The model under review builds one solid part; all positions refer to its coordinate system, in mm. Face numbers are marked on the shaded views. A direction names the side the tool comes from. Coordinates: 2 decimals unless noted, no trailing zeros. Write each loop counter-clockwise with the first axis right and the second up, starting at its lowest first coordinate (ties: lowest second). Pieces come first, ordered by that corner, then holes.
1) Machinability: for the marked faces 1, 2 and 3, which of the approach directions +Z, -Z, +X, -X, +Y, -Y give a long, thin tool a straight path to every point of the face, cutting with its end or side? Answer none if there is none.
2) Add section D-D, the plane y = -7.5. State the section outline as (x, z) points.
3) For P1, Ø5, axis at x = -22.93, y = -0.21, coming from the -Z side; P2, Ø4.5, axis at x = -10.61, y = 10.61, coming from the +Z side; P3, Ø3, axis at x = 20.5, z = 7, coming from the -Y side, all flat-tipped, find the tip position at first contact; note any pin that passes through.
4) Mouldability with a two-part tool opening along X and no side actions: class the marked faces 4, 5, 6 and 7 as released by +X, released by -X, zero draft, split by the parting line, or undercut.
5) Add section B-B, the plane y = 11.5. State the section outline as (x, z) points, then the cut area to 3 significant figures.
6) Add section A-A, the plane x = 0. State the section outline as (y, z) points.
7) Add section C-C, the plane z = 5. Give the number of separate pieces and of enclosed holes in the cut face, then the cut area to 3 significant figures.
8) For line 1 (X direction, y = 14, z = 7.5); line 2 (X direction, y = 0.5, z = 3.5); line 3 (Y direction, x = -13.5, z = 5), list the stretches that pass through material, from the lowest coordinate up.
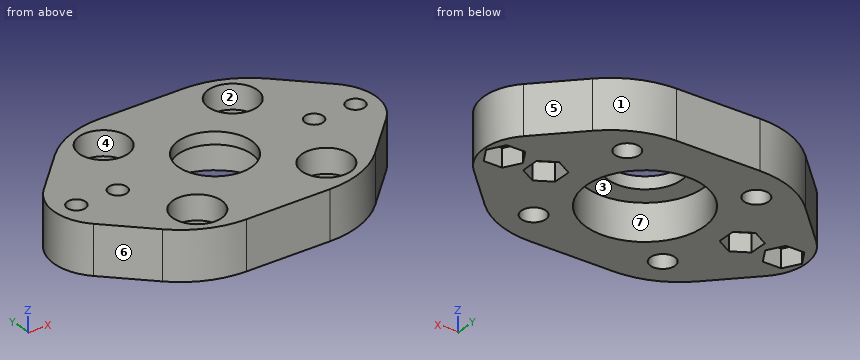
from build123d import *

# Parameters (mm, degrees)
SKETCH1_R           = 2
SKETCH1_R_2         = 9.6
BOSS_EXTRUDE1_DEPTH = 8
SKETCH2_R           = 4
CUT_EXTRUDE1_DEPTH  = 4
SKETCH3_R           = 1.5
CUT_EXTRUDE2_DEPTH  = 10
CUT_EXTRUDE3_DEPTH  = 3
FILLET1_R           = 8
CUT_EXTRUDE4_DEPTH  = 9
FILLET2_R           = 15
SKETCH7_R           = 9.6
SKETCH7_R_2         = 6
BOSS_EXTRUDE2_DEPTH = 2


with BuildPart() as part:
    # Sketch1 → Boss-Extrude1 (new body)
    with BuildSketch(Plane.XY):
        Polygon((-29.69848481, 0), (0, 29.69848481), (29.69848481, 0), (0, -29.69848481), align=None)
        with Locations((10.606601718, 10.606601718)):
            Circle(SKETCH1_R, mode=Mode.SUBTRACT)
        with Locations((10.606601718, -10.606601718)):
            Circle(SKETCH1_R, mode=Mode.SUBTRACT)
        with Locations((-10.606601718, -10.606601718)):
            Circle(SKETCH1_R, mode=Mode.SUBTRACT)
        with Locations((-10.606601718, 10.606601718)):
            Circle(SKETCH1_R, mode=Mode.SUBTRACT)
        Circle(SKETCH1_R_2, mode=Mode.SUBTRACT)
    extrude(amount=BOSS_EXTRUDE1_DEPTH)

    # Sketch2 → Cut-Extrude1 (cut)
    with BuildSketch(Plane.XY.offset(8)):
        with Locations((-10.606601718, 10.606601718)):
            Circle(SKETCH2_R)
        with Locations((10.606601718, 10.606601718)):
            Circle(SKETCH2_R)
        with Locations((10.606601718, -10.606601718)):
            Circle(SKETCH2_R)
        with Locations((-10.606601718, -10.606601718)):
            Circle(SKETCH2_R)
    extrude(amount=-CUT_EXTRUDE1_DEPTH, mode=Mode.SUBTRACT)

    # Sketch3 → Cut-Extrude2 (cut)
    with BuildSketch(Plane.XY.offset(8)):
        with Locations((-22.931196288, -0.213718328)):
            Circle(SKETCH3_R)
        with Locations((-16.131196288, -0.213718328)):
            Circle(SKETCH3_R)
        with Locations((16.131196288, -0.216214782)):
            Circle(SKETCH3_R)
        with Locations((22.931196288, -0.216214782)):
            Circle(SKETCH3_R)
    extrude(amount=-CUT_EXTRUDE2_DEPTH, mode=Mode.SUBTRACT)

    # Sketch4 → Cut-Extrude3 (cut)
    with BuildSketch(Plane(origin=(0, 0, 0), x_dir=(-1, 0, 0), z_dir=(0, 0, -1))):
        Polygon((-24.446740745, 2.408785218), (-25.962285202, -0.216214782), (-24.446740745, -2.841214782), (-21.415651832, -2.841214782), (-19.900107375, -0.216214782), (-21.415651832, 2.408785218), align=None)
        Polygon((-13.506196288, 1.299329674), (-16.131196288, 2.814874131), (-18.756196288, 1.299329674), (-18.756196288, -1.731759239), (-16.131196288, -3.247303696), (-13.506196288, -1.731759239), align=None)
        Polygon((18.756196288, 1.301826129), (16.131196288, 2.817370585), (13.506196288, 1.301826129), (13.506196288, -1.729262785), (16.131196288, -3.244807241), (18.756196288, -1.729262785), align=None)
        Polygon((21.415651832, 2.411281672), (19.900107375, -0.213718328), (21.415651832, -2.838718328), (24.446740745, -2.838718328), (25.962285202, -0.213718328), (24.446740745, 2.411281672), align=None)
    extrude(amount=-CUT_EXTRUDE3_DEPTH, mode=Mode.SUBTRACT)

    # Fillet1
    fillet1_edges = [part.edges().sort_by_distance(p)[0] for p in [
        (-29.69848481, 0, 4),
        (29.69848481, 0, 4),
    ]]
    fillet(fillet1_edges, radius=FILLET1_R)

    # Sketch5 → Cut-Extrude4 (cut, through all)
    with BuildSketch(Plane.XY.offset(8)):
        Polygon((13.091883092, 16.606601718), (0, 29.69848481), (-13.091883092, 16.606601718), align=None)
        Polygon((-13.091883092, -16.606601718), (0, -29.69848481), (13.091883092, -16.606601718), align=None)
    extrude(amount=-CUT_EXTRUDE4_DEPTH, mode=Mode.SUBTRACT)

    # Fillet2
    fillet2_edges = [part.edges().sort_by_distance(p)[0] for p in [
        (13.091883092, 16.606601718, 4),
        (-13.091883092, 16.606601718, 4),
        (-13.091883092, -16.606601718, 4),
        (13.091883092, -16.606601718, 4),
    ]]
    fillet(fillet2_edges, radius=FILLET2_R)

    # Sketch7 → Boss-Extrude2 (add)
    with BuildSketch(Plane.XY.offset(8)):
        Circle(SKETCH7_R)
        Circle(SKETCH7_R_2, mode=Mode.SUBTRACT)
    extrude(amount=-BOSS_EXTRUDE2_DEPTH)


solid = part.part
Geometry results:
1. face 1: +Z, -Z, +X, +Y
1. face 2: +Z
1. face 3: -Z
2. outline: (-22.2, 0) - (-5.99, 0) - (-5.99, 6) - (5.99, 6) - (5.99, 0) - (22.2, 0) - (22.2, 8) - (13.13, 8) - (13.13, 4) - (8.09, 4) - (8.09, 8) - (-8.09, 8) - (-8.09, 4) - (-13.13, 4) - (-13.13, 8) - (-22.2, 8) - close
3. P1: stops at z = 3
3. P2: stops at z = 4
3. P3: stops at y = -10.7
4. face 4: undercut
4. face 5: released by +X
4. face 6: released by -X
4. face 7: undercut
5. outline: (-18.2, 0) - (-12.4, 0) - (-12.4, 4) - (-14.51, 4) - (-14.51, 8) - (-18.2, 8) - close; (-8.82, 0) - (8.82, 0) - (8.82, 4) - (6.71, 4) - (6.71, 8) - (-6.71, 8) - (-6.71, 4) - (-8.82, 4) - close; (12.4, 0) - (18.2, 0) - (18.2, 8) - (14.51, 8) - (14.51, 4) - (12.4, 4) - close
5. area: 200 mm2
6. outline: (-16.61, 0) - (-9.6, 0) - (-9.6, 6) - (-6, 6) - (-6, 8) - (-16.61, 8) - close; (6, 6) - (9.6, 6) - (9.6, 0) - (16.61, 0) - (16.61, 8) - (6, 8) - close
7. separate pieces: 1
7. enclosed holes: 9
7. area: 856 mm2
8. line 1: x = -15.33 to -12.72, -8.49 to 8.49, 12.72 to 15.33
8. line 2: x = -26.37 to -24.25, -21.61 to -17.45, -14.81 to -9.59, 9.59 to 14.81, 17.45 to 21.61, 24.25 to 26.37
8. line 3: y = -15.07 to -13.37, -7.84 to 7.84, 13.37 to 15.07
